Design review of the part built by this model. Coordinates are the model's own, in mm. Face numbers are marked on the shaded views. Round coordinates to 2 decimals unless told otherwise and drop trailing zeros. Order: outer loops, then holes, each group sorted by start corner. A loop starts at its lowest first (then second) coordinate and runs counter-clockwise, first axis right, second up.
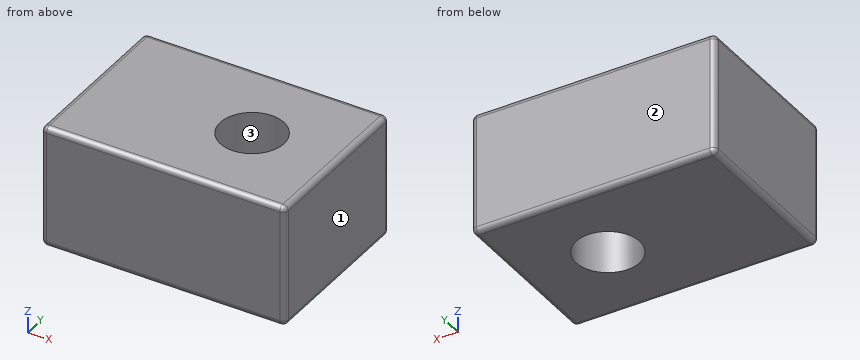
Autodesk Inventor part; units mm, degrees
ref_plane "YZ Plane" through (0, 0, 0) normal (1, 0, 0) x (0, 1, 0)
ref_plane "XZ Plane" through (0, 0, 0) normal (0, 1, 0) x (-1, 0, 0)
ref_plane "XY Plane" through (0, 0, 0) normal (0, 0, 1) x (1, 0, 0)
sketch "Sketch1" plane through (0, 0, 0) normal (0, 0, 1) x (1, 0, 0)
  line L0 (-11.5, 8) -> (11.5, 8)
  line L1 (11.5, 8) -> (11.5, -8)
  line L2 (11.5, -8) -> (-11.5, -8)
  line L3 (-11.5, -8) -> (-11.5, 8)
  circle A0 centre (3.5, 0) radius 3
  point P0 (0, 0)
  point P1 (0, 8)
  point P2 (-11.5, 0)
  dimension "d0" = 23
  dimension "d2" = 16
  dimension "d3" = 6
  dimension "d4" = 8
extrude "Extrusion1" add sketch "Sketch1" along normal blind 11.5
fillet "Fillet1" radius 0.5 12 edges at (0, 8, 11.5) (-11.5, 0, 11.5) (0, -8, 11.5) (11.5, 0, 11.5) (0, 8, 0) (-11.5, 8, 5.75) (11.5, 8, 5.75) (0, -8, 0) (11.5, -8, 5.75) (-11.5, -8, 5.75) (11.5, 0, 0) (-11.5, 0, 0)
properties part number "heat block"
1) Take a section at A-A on x = 3.5. Give the boundary of the cut face in (y, z), plus the area to 3 significant figures.
Results:
outline: (-8, 0.5) arc R0.5 ccw to (-7.5, 0) - (-3, 0) - (-3, 11.5) - (-7.5, 11.5) arc R0.5 ccw to (-8, 11) - close; (3, 0) - (7.5, 0) arc R0.5 ccw to (8, 0.5) - (8, 11) arc R0.5 ccw to (7.5, 11.5) - (3, 11.5) - close
area: 115 mm2
2) To check wall thickness, follow line 1 along Y through (x, z) = (3.5, 5); line 2 along X through (y, z) = (1.5, 8.5); line 3 along X through (y, z) = (-1, 1.5). State the ranges of each line that lie inside material, in increasing order.
Results:
line 1: y = -8 to -3, 3 to 8
line 2: x = -11.5 to 0.9, 6.1 to 11.5
line 3: x = -11.5 to 0.67, 6.33 to 11.5
3) The part is to be moulded in two halves that separate along X. For the marked faces 1, 2 and 3, say which applies: released by +X, released by -X, zero draft, split by the parting line, or undercut.
Results:
face 1: released by +X
face 2: zero draft
face 3: undercut
4) Take a section at C-C on y = 0. Give the boundary of the cut face in (x, z), plus the area to 3 significant figures.
Results:
outline: (-11.5, 0.5) arc R0.5 ccw to (-11, 0) - (0.5, 0) - (0.5, 11.5) - (-11, 11.5) arc R0.5 ccw to (-11.5, 11) - close; (6.5, 0) - (11, 0) arc R0.5 ccw to (11.5, 0.5) - (11.5, 11) arc R0.5 ccw to (11, 11.5) - (6.5, 11.5) - close
area: 195 mm2
5) Take a section at B-B on z = 10.5. Give the boundary of the cut face in (x, y), plus the area to 3 significant figures.
Results:
outline: (-11.5, -7.5) arc R0.5 ccw to (-11, -8) - (11, -8) arc R0.5 ccw to (11.5, -7.5) - (11.5, 7.5) arc R0.5 ccw to (11, 8) - (-11, 8) arc R0.5 ccw to (-11.5, 7.5) - close; hole circle Ø6 at (3.5, 0)
area: 340 mm2
